from build123d import *

# Parameters (mm, degrees)
F0_W     = 936.625
F0_H     = 1393.825
F1_DEPTH = 19.05
F2_W     = 92.075
F2_H     = 92.075
F3_DEPTH = 19.051
F4_W     = 41.275
F4_H     = 434.975
F5_DEPTH = 19.051


with BuildPart() as f1:
    # F0 (on Top) → F1 (new body)
    with BuildSketch(Plane.XY):
        Rectangle(F0_W, F0_H)
    extrude(amount=F1_DEPTH)

    # F2 (on face) → F3 (cut, through all)
    with BuildSketch(Plane.XY.offset(19.05)):
        with Locations((-422.275, 650.875)):
            Rectangle(F2_W, F2_H)
        with Locations((422.275, 650.875)):
            Rectangle(F2_W, F2_H)
        with Locations((422.275, -650.875)):
            Rectangle(F2_W, F2_H)
        with Locations((-422.275, -650.875)):
            Rectangle(F2_W, F2_H)
    extrude(amount=-F3_DEPTH, mode=Mode.SUBTRACT)

    # F4 (on face) → F5 (cut, through all)
    with BuildSketch(Plane.XY.offset(19.05)):
        with Locations((-447.675, 387.35)):
            Rectangle(F4_W, F4_H)
    extrude(amount=-F5_DEPTH, mode=Mode.SUBTRACT)


solid = f1.part
For this review, take the finished solid that the model builds, in its own axes (mm). Give positions to 0.01 mm unless a question says otherwise; leave off trailing zeros. Loops run counter-clockwise (first coordinate to the right, second up) from the corner with the lowest first, then second, coordinate; pieces in that order, holes last. Notation, with made-up numbers: M 33,63 L 42,63 A24 cw 42,86 Z; hole C 69.5,12 d2. An arc over 180 degrees is marked long. Answer as a JSON object with one key per item and string values. Group by question number.
Q1. For probe 1 along X at (y, z) = (443.5, 12.75); probe 2 along X at (y, z) = (613, 4.5), list the stretches that pass through material, from the lowest coordinate up. Write a range as [from, to].
Q2. Insertion check: P1, Ø5.5, axis at x = -442.5, z = 13.5, coming from the +Y side; P2, Ø9.5, axis at x = -426.5, z = 7, coming from the -Y side; P3, Ø9.5, axis at y = -640.5, z = 10.5, coming from the +X side; P4, Ø8, axis at x = 120.5, y = 28.5, coming from the -Z side. Each pin has a flat end and moves straight along its axis. Give the tip position at first contact, or say it passes through.
Q3. Add section A-A on z = 10.5. Give the boundary of the cut face in (x, y).
Q4. Add section B-B on y = 446. Give the boundary of the cut face in (x, z), and give its area (3 significant figures).
Checked values:
{
 "1": {"probe 1": "[-427.04, 468.31]", "probe 2": "[-376.24, 376.24]"},
 "2": {"P1": "y = 169.86", "P2": "y = -604.84", "P3": "x = 376.24", "P4": "z = 0"},
 "3": {"outline": "M -468.31,-604.84 L -376.24,-604.84 L -376.24,-696.91 L 376.24,-696.91 L 376.24,-604.84 L 468.31,-604.84 L 468.31,604.84 L 376.24,604.84 L 376.24,696.91 L -376.24,696.91 L -376.24,604.84 L -427.04,604.84 L -427.04,169.86 L -468.31,169.86 Z"},
 "4": {"outline": "M -427.04,0 L 468.31,0 L 468.31,19.05 L -427.04,19.05 Z", "area": "17,100 mm²"}
}
